Could you check a few things on this model? Use its own coordinates, in mm. A direction names the side the tool comes from. Coordinates: 2 decimals unless noted, no trailing zeros. Loops run counter-clockwise (first coordinate to the right, second up) from the corner with the lowest first, then second, coordinate; pieces in that order, holes last. Notation, with made-up numbers: (22.25, -20.75) - (41.25, -20.75) arc R30 ccw to (41.25, 8.25) - close; hole circle Ø9 at (-32, -18). An arc over 180 degrees is marked (long way). One line per item, written item: value. Start each with the question number.
(1) If we mould it in two halves opening along Z, with no side actions, what happens to faces 3 (the face through (-3, -10, -135)), 4 (the face through (-65.594, -10.874, 88.487)), 5 (the face through (-53, 0, 118))? For each: pulls with the +Z half, pulls with the -Z half, needs draft (parallel to the pull), parting line crosses it, or undercut.
(2) On a 3-axis mill with a long thin cutter (end or side, diameter ignored), from which of +Z, -Z, +X, -X, +Y, -Y can I reach the whole of each face in a straight line? I mean faces 1 (the face through (143.215, -10.874, 85.713)), 2 (the face through (-108.986, -1.014, 109.297)). Say none if no direction works.
(3) I'm going to push flat-ended pins straight in: P1, Ø7.5, axis at x = -124, z = 65, coming from the -Y side; P2, Ø4, axis at x = -86, z = 75, coming from the +Y side; P3, Ø3.5, axis at x = -125, z = -104.5, coming from the -Y side; P4, Ø4.5, axis at x = 57.5, z = 18.5, coming from the +Y side. Where does each tip first touch, or does it pass through?
(4) If we section it at A-A on x = 35: Write out the boundary of the cut face in (y, z), then the cut area to 3 significant figures.
(5) If I drill on line 1 along X through (y, z) = (-12.5, -88); line 2 along X through (y, z) = (-10.25, -28); line 3 along X through (y, z) = (-12.75, -5), over which ranges is the centre line in solid material (lowest first)? Write a range as from..to.
```python
from build123d import *

# Parameters (mm, degrees)
SKETCH_1_W          = 450
SKETCH_1_H          = 270
EXTRUDE_1_DEPTH     = 20
SKETCH_1_3_W        = 300
SKETCH_1_3_H        = 245
CUT_EXTRUDE_1_DEPTH = 2
CUT_EXTRUDE_2_REACH = 265.154
SKETCH_1_4_R        = 22
SKETCH_1_4_R_2      = 13.5
FILLET_1_R          = 20
SKETCH_3_R          = 2.1
CUT_EXTRUDE_3_DEPTH = 10
SKETCH_4_R          = 3.35
CUT_EXTRUDE_4_DEPTH = 12


with BuildPart() as part:
    # Sketch 1 → Extrude 1 (new body)
    with BuildSketch(Plane(origin=(0, 0, 0), x_dir=(1, 0, 0), z_dir=(0, 1, 0))):
        Rectangle(SKETCH_1_W, SKETCH_1_H)
    extrude(amount=-EXTRUDE_1_DEPTH)

    # Sketch 1_3 → Cut-Extrude 1 (cut)
    with BuildSketch(Plane(origin=(0, 0, 0), x_dir=(1, 0, 0), z_dir=(0, 1, 0))):
        with Locations((35, 7.5)):
            Rectangle(SKETCH_1_3_W, SKETCH_1_3_H)
    extrude(amount=-CUT_EXTRUDE_1_DEPTH, mode=Mode.SUBTRACT)

    # Sketch 1_4 → Cut-Extrude 2 (cut, up to next)
    with BuildSketch(Plane(origin=(0, 0, 0), x_dir=(1, 0, 0), z_dir=(0, 1, 0)), mode=Mode.PRIVATE) as cut_extrude_2_sk1:
        with Locations(Location((-65, 90, 0), (0, 0, 90))):
            Circle(SKETCH_1_4_R)
    cut_extrude_2_tool1 = extrude(cut_extrude_2_sk1.sketch, amount=-CUT_EXTRUDE_2_REACH, mode=Mode.PRIVATE) & part.part
    # Sketch 1_4 → Cut-Extrude 2 (cut, up to next)
    with BuildSketch(Plane(origin=(0, 0, 0), x_dir=(1, 0, 0), z_dir=(0, 1, 0)), mode=Mode.PRIVATE) as cut_extrude_2_sk2:
        with Locations(Location((35, 90, 0), (0, 0, 90))):
            Circle(SKETCH_1_4_R)
    cut_extrude_2_tool2 = extrude(cut_extrude_2_sk2.sketch, amount=-CUT_EXTRUDE_2_REACH, mode=Mode.PRIVATE) & part.part
    # Sketch 1_4 → Cut-Extrude 2 (cut, up to next)
    with BuildSketch(Plane(origin=(0, 0, 0), x_dir=(1, 0, 0), z_dir=(0, 1, 0)), mode=Mode.PRIVATE) as cut_extrude_2_sk3:
        with Locations(Location((135, 90, 0), (0, 0, 90))):
            Circle(SKETCH_1_4_R)
    cut_extrude_2_tool3 = extrude(cut_extrude_2_sk3.sketch, amount=-CUT_EXTRUDE_2_REACH, mode=Mode.PRIVATE) & part.part
    # Sketch 1_4 → Cut-Extrude 2 (cut, up to next)
    with BuildSketch(Plane(origin=(0, 0, 0), x_dir=(1, 0, 0), z_dir=(0, 1, 0)), mode=Mode.PRIVATE) as cut_extrude_2_sk4:
        with Locations(Location((135, 5, 0), (0, 0, 90))):
            Circle(SKETCH_1_4_R)
    cut_extrude_2_tool4 = extrude(cut_extrude_2_sk4.sketch, amount=-CUT_EXTRUDE_2_REACH, mode=Mode.PRIVATE) & part.part
    # Sketch 1_4 → Cut-Extrude 2 (cut, up to next)
    with BuildSketch(Plane(origin=(0, 0, 0), x_dir=(1, 0, 0), z_dir=(0, 1, 0)), mode=Mode.PRIVATE) as cut_extrude_2_sk5:
        with Locations(Location((35, 5, 0), (0, 0, 90))):
            Circle(SKETCH_1_4_R)
    cut_extrude_2_tool5 = extrude(cut_extrude_2_sk5.sketch, amount=-CUT_EXTRUDE_2_REACH, mode=Mode.PRIVATE) & part.part
    # Sketch 1_4 → Cut-Extrude 2 (cut, up to next)
    with BuildSketch(Plane(origin=(0, 0, 0), x_dir=(1, 0, 0), z_dir=(0, 1, 0)), mode=Mode.PRIVATE) as cut_extrude_2_sk6:
        with Locations(Location((-65, 5, 0), (0, 0, 90))):
            Circle(SKETCH_1_4_R)
    cut_extrude_2_tool6 = extrude(cut_extrude_2_sk6.sketch, amount=-CUT_EXTRUDE_2_REACH, mode=Mode.PRIVATE) & part.part
    # Sketch 1_4 → Cut-Extrude 2 (cut, up to next)
    with BuildSketch(Plane(origin=(0, 0, 0), x_dir=(1, 0, 0), z_dir=(0, 1, 0)), mode=Mode.PRIVATE) as cut_extrude_2_sk7:
        with Locations(Location((-65, -75, 0), (0, 0, 90))):
            Circle(SKETCH_1_4_R_2)
    cut_extrude_2_tool7 = extrude(cut_extrude_2_sk7.sketch, amount=-CUT_EXTRUDE_2_REACH, mode=Mode.PRIVATE) & part.part
    # Sketch 1_4 → Cut-Extrude 2 (cut, up to next)
    with BuildSketch(Plane(origin=(0, 0, 0), x_dir=(1, 0, 0), z_dir=(0, 1, 0)), mode=Mode.PRIVATE) as cut_extrude_2_sk8:
        with Locations(Location((35, -75, 0), (0, 0, 90))):
            Circle(SKETCH_1_4_R_2)
    cut_extrude_2_tool8 = extrude(cut_extrude_2_sk8.sketch, amount=-CUT_EXTRUDE_2_REACH, mode=Mode.PRIVATE) & part.part
    # Sketch 1_4 → Cut-Extrude 2 (cut, up to next)
    with BuildSketch(Plane(origin=(0, 0, 0), x_dir=(1, 0, 0), z_dir=(0, 1, 0)), mode=Mode.PRIVATE) as cut_extrude_2_sk9:
        with Locations(Location((135, -75, 0), (0, 0, 90))):
            Circle(SKETCH_1_4_R_2)
    cut_extrude_2_tool9 = extrude(cut_extrude_2_sk9.sketch, amount=-CUT_EXTRUDE_2_REACH, mode=Mode.PRIVATE) & part.part
    add(cut_extrude_2_tool1.solids().sort_by_distance((-65, 0, -90))[0], mode=Mode.SUBTRACT)
    add(cut_extrude_2_tool2.solids().sort_by_distance((35, 0, -90))[0], mode=Mode.SUBTRACT)
    add(cut_extrude_2_tool3.solids().sort_by_distance((135, 0, -90))[0], mode=Mode.SUBTRACT)
    add(cut_extrude_2_tool4.solids().sort_by_distance((135, 0, -5))[0], mode=Mode.SUBTRACT)
    add(cut_extrude_2_tool5.solids().sort_by_distance((35, 0, -5))[0], mode=Mode.SUBTRACT)
    add(cut_extrude_2_tool6.solids().sort_by_distance((-65, 0, -5))[0], mode=Mode.SUBTRACT)
    add(cut_extrude_2_tool7.solids().sort_by_distance((-65, 0, 75))[0], mode=Mode.SUBTRACT)
    add(cut_extrude_2_tool8.solids().sort_by_distance((35, 0, 75))[0], mode=Mode.SUBTRACT)
    add(cut_extrude_2_tool9.solids().sort_by_distance((135, 0, 75))[0], mode=Mode.SUBTRACT)

    # Fillet 1
    fillet_1_edges = [part.edges().sort_by_distance(p)[0] for p in [
        (-115, -1, -130),
        (185, -1, -130),
        (185, -1, 115),
        (-115, -1, 115),
    ]]
    fillet(fillet_1_edges, radius=FILLET_1_R)

    # Sketch 3 → Cut-Extrude 3 (cut)
    with BuildSketch(Plane(origin=(0, -2, 0), x_dir=(1, 0, 0), z_dir=(0, 1, 0))):
        with Locations(Location((-41.665476221, 66.665476221, 0), (0, 0, 270))):
            Circle(SKETCH_3_R)
        with Locations(Location((-88.334523779, 113.334523779, 0), (0, 0, 270))):
            Circle(SKETCH_3_R)
        with Locations(Location((58.334523779, 66.665476221, 0), (0, 0, 270))):
            Circle(SKETCH_3_R)
        with Locations(Location((11.665476221, 113.334523779, 0), (0, 0, 270))):
            Circle(SKETCH_3_R)
        with Locations(Location((158.334523779, 66.665476221, 0), (0, 0, 270))):
            Circle(SKETCH_3_R)
        with Locations(Location((111.665476221, 113.334523779, 0), (0, 0, 270))):
            Circle(SKETCH_3_R)
        with Locations(Location((58.334523779, -18.334523779, 0), (0, 0, 270))):
            Circle(SKETCH_3_R)
        with Locations(Location((11.665476221, 28.334523779, 0), (0, 0, 270))):
            Circle(SKETCH_3_R)
        with Locations(Location((158.334523779, -18.334523779, 0), (0, 0, 270))):
            Circle(SKETCH_3_R)
        with Locations(Location((111.665476221, 28.334523779, 0), (0, 0, 270))):
            Circle(SKETCH_3_R)
        with Locations(Location((-41.665476221, -18.334523779, 0), (0, 0, 270))):
            Circle(SKETCH_3_R)
        with Locations(Location((-88.334523779, 28.334523779, 0), (0, 0, 270))):
            Circle(SKETCH_3_R)
        with Locations(Location((-86, -75, 0), (0, 0, 270))):
            Circle(SKETCH_3_R)
        with Locations(Location((-44, -75, 0), (0, 0, 270))):
            Circle(SKETCH_3_R)
        with Locations(Location((14, -75, 0), (0, 0, 270))):
            Circle(SKETCH_3_R)
        with Locations(Location((56, -75, 0), (0, 0, 270))):
            Circle(SKETCH_3_R)
        with Locations(Location((114, -75, 0), (0, 0, 270))):
            Circle(SKETCH_3_R)
        with Locations(Location((156, -75, 0), (0, 0, 270))):
            Circle(SKETCH_3_R)
    extrude(amount=-CUT_EXTRUDE_3_DEPTH, mode=Mode.SUBTRACT)

    # Sketch 4 → Cut-Extrude 4 (cut)
    with BuildSketch(Plane.XZ.offset(20)):
        with Locations(Location((-124, 65, 0), (0, 0, 270))):
            Circle(SKETCH_4_R)
        with Locations(Location((210, 65, 0), (0, 0, 270))):
            Circle(SKETCH_4_R)
        with Locations(Location((210, 30, 0), (0, 0, 270))):
            Circle(SKETCH_4_R)
        with Locations(Location((210, -70, 0), (0, 0, 270))):
            Circle(SKETCH_4_R)
        with Locations(Location((-174, -70, 0), (0, 0, 270))):
            Circle(SKETCH_4_R)
        with Locations(Location((-174, 30, 0), (0, 0, 270))):
            Circle(SKETCH_4_R)
        with Locations(Location((-124, -105, 0), (0, 0, 270))):
            Circle(SKETCH_4_R)
        with Locations(Location((100, -105, 0), (0, 0, 270))):
            Circle(SKETCH_4_R)
        with Locations(Location((100, -5, 0), (0, 0, 270))):
            Circle(SKETCH_4_R)
    extrude(amount=-CUT_EXTRUDE_4_DEPTH, mode=Mode.SUBTRACT)


solid = part.part
```
Values:
1. face 3: pulls with the -Z half
1. face 4: undercut
1. face 5: needs draft
2. face 1: +Y, -Y
2. face 2: +Y
3. P1: stops at y = -20
3. P2: stops at y = -12
3. P3: stops at y = -8
3. P4: stops at y = -2
4. outline: (-20, -135) - (0, -135) - (0, -130) - (-2, -130) - (-2, -112) - (-20, -112) - close; (-20, -68) - (-2, -68) - (-2, -27) - (-20, -27) - close; (-20, 17) - (-2, 17) - (-2, 61.5) - (-20, 61.5) - close; (-20, 88.5) - (-2, 88.5) - (-2, 115) - (0, 115) - (0, 135) - (-20, 135) - close
4. area: 2,840 mm2
5. line 1: x = -225..-86.91, -43.09..13.09, 56.91..113.09, 156.91..225
5. line 2: x = -225..-90.41, -86.26..9.59, 13.74..109.59, 113.74..225
5. line 3: x = -225..-87, -43..13, 57..96.65, 103.35..113, 157..225
